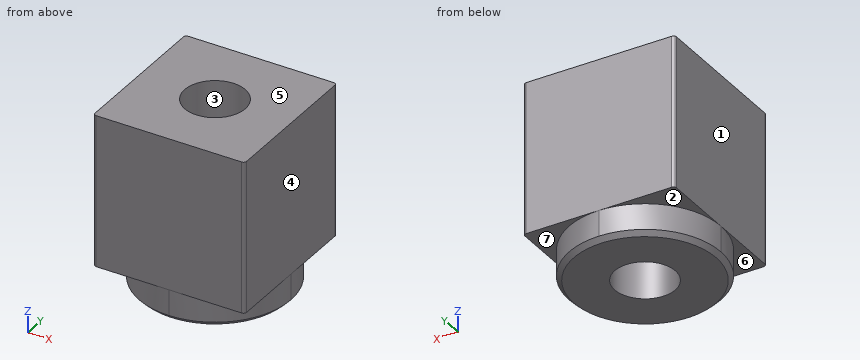
from build123d import *

# Parameters (mm, degrees)
F0_R     = 2
F1_DEPTH = 10
F2_DEPTH = 2
F4_R     = 0.2


# Not quite as in the source:
# - a fillet or chamfer that OpenCascade refuses, or shapes differently, is made with other operations: its cross-section is extruded or revolved along the edge and cut away or added


with BuildPart() as f1:
    # F0 (on Top) → F1 (new body)
    with BuildSketch(Plane.XY):
        with BuildLine():
            Line((5, 0), (5, 5))
            Line((5, 5), (0, 5))
            ThreePointArc((0, 5), (3.5355339059, 3.5355339059), (5, 0))
        make_face()
        with BuildLine():
            ThreePointArc((-5, 0), (-3.5355339059, 3.5355339059), (0, 5))
            Line((0, 5), (-5, 5))
            Line((-5, 5), (-5, 0))
        make_face()
        with BuildLine():
            ThreePointArc((5, 0), (3.5355339059, 3.5355339059), (0, 5))
            ThreePointArc((0, 5), (-3.5355339059, 3.5355339059), (-5, 0))
            ThreePointArc((-5, 0), (-3.5355339059, -3.5355339059), (0, -5))
            ThreePointArc((0, -5), (3.5355339059, -3.5355339059), (5, 0))
        make_face()
        Circle(F0_R, mode=Mode.SUBTRACT)
        with BuildLine():
            Line((5, -5), (5, 0))
            ThreePointArc((5, 0), (3.5355339059, -3.5355339059), (0, -5))
            Line((0, -5), (5, -5))
        make_face()
        with BuildLine():
            ThreePointArc((0, -5), (-3.5355339059, -3.5355339059), (-5, 0))
            Line((-5, 0), (-5, -5))
            Line((-5, -5), (0, -5))
        make_face()
    extrude(amount=F1_DEPTH)

    # F0 (on Top) → F2 (join)
    with BuildSketch(Plane.XY):
        with BuildLine():
            ThreePointArc((5, 0), (3.5355339059, 3.5355339059), (0, 5))
            ThreePointArc((0, 5), (-3.5355339059, 3.5355339059), (-5, 0))
            ThreePointArc((-5, 0), (-3.5355339059, -3.5355339059), (0, -5))
            ThreePointArc((0, -5), (3.5355339059, -3.5355339059), (5, 0))
        make_face()
        Circle(F0_R, mode=Mode.SUBTRACT)
    extrude(amount=-F2_DEPTH)

    # F3: chamfer of 0.3 on 1 edges, made by hand

    # F3_s1 → F3_t2 (revolve, cut)
    with BuildSketch(Plane.XZ):
        Polygon((-4.7, -2), (-5, -1.7), (-5, -2), align=None)
    revolve(axis=Axis((0, 0, -2), (0, 0, 1)), mode=Mode.SUBTRACT)

    # F4
    f4_edges = [f1.edges().sort_by_distance(p)[0] for p in [
        (5, 5, 5),
        (5, -5, 5),
        (-5, 5, 5),
        (-5, -5, 5),
    ]]
    fillet(f4_edges, radius=F4_R)


solid = f1.part
The model under review builds one solid part; all positions refer to its coordinate system, in mm. Face numbers are marked on the shaded views. A direction names the side the tool comes from. Coordinates: 2 decimals unless noted, no trailing zeros. Order: outer loops, then holes, each group sorted by start corner. A loop starts at its lowest first (then second) coordinate and runs counter-clockwise, first axis right, second up. Notation, with made-up numbers: (-33, -33.75) -> (-7, -33.75) arc R12 ccw to (-7, -20.75) -> close; hole circle Ø8 at (72, 48). An arc over 180 degrees is marked (long way). Answer in a Markdown table with one row per item.
(1) Insertion check: pin 1 (3.5 mm diameter, centred on x = 0, y = 0, fed in from +Z). The pin has a flat end and moves straight along its axis. Give the tip position at first contact, or say it passes through.
Answers:
| item | result |
|---|---|
| pin 1 | through |
(2) Consider section B-B (z = -0.5). Write out the cut boundary in (x, y), plus the area to 3 significant figures.
Answers:
| item | result |
|---|---|
| outline | circle Ø10 at (0, 0); hole circle Ø4 at (0, 0) |
| area | 66.0 mm² |
(3) Consider section A-A (z = 9.25). Write out the cut boundary in (x, y), plus the area to 3 significant figures.
Answers:
| item | result |
|---|---|
| outline | (-5, -4.8) arc R0.2 ccw to (-4.8, -5) -> (4.8, -5) arc R0.2 ccw to (5, -4.8) -> (5, 4.8) arc R0.2 ccw to (4.8, 5) -> (-4.8, 5) arc R0.2 ccw to (-5, 4.8) -> close; hole circle Ø4 at (0, 0) |
| area | 87.4 mm² |
(4) Machinability: for the marked faces 5, 6 and 7, which of the approach directions +Z, -Z, +X, -X, +Y, -Y give a long, thin tool a straight path to every point of the face, cutting with its end or side? Answer none if there is none.
Answers:
| item | result |
|---|---|
| face 5 | +Z, +X, -X, +Y, -Y |
| face 6 | -Z, -X, -Y |
| face 7 | -Z, +X, +Y |
(5) The part is to be moulded in two halves that separate along X. For the marked faces 1, 2, 3 and 4, say which applies: +X half, -X half, draft (parallel to the pull), parting line (faces both ways), or undercut.
Answers:
| item | result |
|---|---|
| face 1 | -X half |
| face 2 | draft |
| face 3 | undercut |
| face 4 | +X half |
(6) Wall thickness on line 1 along Y through (x, z) = (0, 3); line 2 along Y through (x, z) = (-1, 2.75): over which ranges is each line inside the solid? List them lowest first.
Answers:
| item | result |
|---|---|
| line 1 | -5 to -2, 2 to 5 |
| line 2 | -5 to -1.73, 1.73 to 5 |
